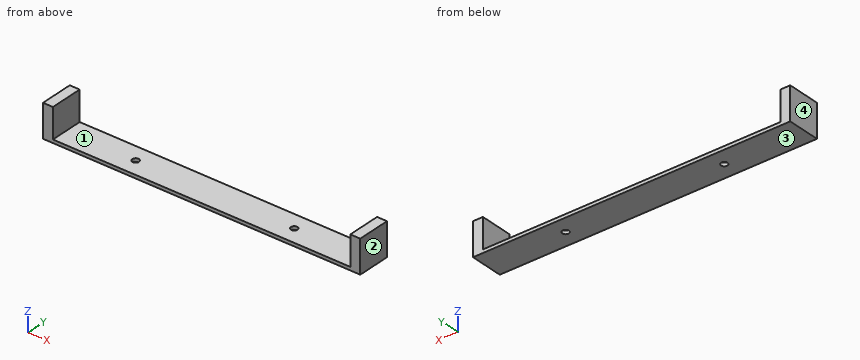
```python
from build123d import *

# Parameters (mm, degrees)
SKETCH_W     = 90
SKETCH_H     = 10
SKETCH_R     = 1
PAD_DEPTH    = 1
SKETCH001_W  = 3
SKETCH001_H  = 10
PAD001_DEPTH = 10


with BuildPart() as part:
    # Sketch → Pad (new body)
    with BuildSketch(Plane.XY):
        Rectangle(SKETCH_W, SKETCH_H)
        with Locations((-24, 0)):
            Circle(SKETCH_R, mode=Mode.SUBTRACT)
        with Locations((24, 0)):
            Circle(SKETCH_R, mode=Mode.SUBTRACT)
    extrude(amount=PAD_DEPTH)

    # Sketch001 → Pad001 (join)
    with BuildSketch(Plane.XY):
        with Locations((-46.5, 0)):
            Rectangle(SKETCH001_W, SKETCH001_H)
        with Locations((46.5, 0)):
            Rectangle(SKETCH001_W, SKETCH001_H)
    extrude(amount=PAD001_DEPTH)


solid = part.part
```
Read the model definition and answer for the solid it produces. Units are mm, in the model's axes. Face numbers are marked on the shaded views. Give positions to 0.01 mm unless a question says otherwise; leave off trailing zeros. Write each loop counter-clockwise with the first axis right and the second up, starting at its lowest first coordinate (ties: lowest second). Pieces come first, ordered by that corner, then holes. Notation, with made-up numbers: (-14, 86.25) -> (-5, 86.25) arc R22 ccw to (-5, 115.25) -> close; hole circle Ø4 at (40, 11.5). An arc over 180 degrees is marked (long way). Answer in a Markdown table with one row per item.
1) This flat-tipped pin is pushed along its axis until it touches: pin 1 Ø4 at (x, y) = (-6.5, -4) entering from +Z. Where does it stop, or does it pass through?
Results list:
| item | result |
|---|---|
| pin 1 | z = 1 |
2) Section B-B on z = 7 is taken. Give the vertices of the cut face in (x, y), plus the area to 3 significant figures.
Results list:
| item | result |
|---|---|
| outline | (-48, -5) -> (-45, -5) -> (-45, 5) -> (-48, 5) -> close; (45, -5) -> (48, -5) -> (48, 5) -> (45, 5) -> close |
| area | 60.0 mm^2 |
3) Section C-C on y = 0 is taken. Give the vertices of the cut face in (x, z).
Results list:
| item | result |
|---|---|
| outline | (-48, 0) -> (-25, 0) -> (-25, 1) -> (-45, 1) -> (-45, 10) -> (-48, 10) -> close; (-23, 0) -> (23, 0) -> (23, 1) -> (-23, 1) -> close; (25, 0) -> (48, 0) -> (48, 10) -> (45, 10) -> (45, 1) -> (25, 1) -> close |
4) Straight lines are drawn through the part: line 1 (X direction, y = -2, z = 8.75); line 2 (Y direction, x = -24, z = 0.85); line 3 (Z direction, x = -7, y = 1). For each, find the intervals that lie inside material, in ascending order. Write a range as [from, to].
Results list:
| item | result |
|---|---|
| line 1 | [-48, -45], [45, 48] |
| line 2 | [-5, -1], [1, 5] |
| line 3 | [0, 1] |
5) Section A-A on x = -24 is taken. Give the vertices of the cut face in (y, z).
Results list:
| item | result |
|---|---|
| outline | (-5, 0) -> (-1, 0) -> (-1, 1) -> (-5, 1) -> close; (1, 0) -> (5, 0) -> (5, 1) -> (1, 1) -> close |
6) Determine the mould class of the marked faces 1, 2, 3 and 4 for opening direction X: released by +X, released by -X, zero draft, split by the parting line, or undercut.
Results list:
| item | result |
|---|---|
| face 1 | undercut |
| face 2 | released by +X |
| face 3 | zero draft |
| face 4 | released by -X |
7) Section D-D on x = -41.5 is taken. Give the vertices of the cut face in (y, z).
Results list:
| item | result |
|---|---|
| outline | (-5, 0) -> (5, 0) -> (5, 1) -> (-5, 1) -> close |
